Build history of the part. All positions in model axes, mm. Coordinates: 2 decimals unless noted, no trailing zeros. Order: outer loops, then holes, each group sorted by start corner. A loop starts at its lowest first (then second) coordinate and runs counter-clockwise, first axis right, second up. Notation, with made-up numbers: (-16, -36) - (-2, -36) arc R36 cw to (-2, -2) - close; hole circle Ø10 at (-12.5, -4). An arc over 180 degrees is marked (long way). One line per item, written item: value.
from build123d import *

# Parameters (mm, degrees)
SKETCH1_W           = 40.64
SKETCH1_H           = 50.673
SKETCH1_R           = 15.875
BOSS_EXTRUDE1_DEPTH = 6.35
CUT_EXTRUDE1_REACH  = 35.093
SKETCH2_R           = 2.665
FILLET1_R           = 2.54


with BuildPart() as part:
    # Sketch1 → Boss-Extrude1 (new body)
    with BuildSketch(Plane(origin=(0, 0, 0), x_dir=(1, 0, 0), z_dir=(0, 1, 0))):
        Rectangle(SKETCH1_W, SKETCH1_H)
        with Locations(Location((0, 0, 0), (0, 0, 270))):
            Circle(SKETCH1_R, mode=Mode.SUBTRACT)
    extrude(amount=BOSS_EXTRUDE1_DEPTH)

    # Sketch2 → Cut-Extrude1 (cut, up to next)
    with BuildSketch(Plane(origin=(0, 6.35, 0), x_dir=(1, 0, 0), z_dir=(0, 1, 0)), mode=Mode.PRIVATE) as cut_extrude1_sk1:
        with Locations(Location((-15.32, 20.3365, 0), (0, 0, 270))):
            Circle(SKETCH2_R)
    cut_extrude1_tool1 = extrude(cut_extrude1_sk1.sketch, amount=-CUT_EXTRUDE1_REACH, mode=Mode.PRIVATE) & part.part
    # Sketch2 → Cut-Extrude1 (cut, up to next)
    with BuildSketch(Plane(origin=(0, 6.35, 0), x_dir=(1, 0, 0), z_dir=(0, 1, 0)), mode=Mode.PRIVATE) as cut_extrude1_sk2:
        with Locations(Location((15.32, 20.3365, 0), (0, 0, 270))):
            Circle(SKETCH2_R)
    cut_extrude1_tool2 = extrude(cut_extrude1_sk2.sketch, amount=-CUT_EXTRUDE1_REACH, mode=Mode.PRIVATE) & part.part
    # Sketch2 → Cut-Extrude1 (cut, up to next)
    with BuildSketch(Plane(origin=(0, 6.35, 0), x_dir=(1, 0, 0), z_dir=(0, 1, 0)), mode=Mode.PRIVATE) as cut_extrude1_sk3:
        with Locations(Location((15.32, -20.3365, 0), (0, 0, 270))):
            Circle(SKETCH2_R)
    cut_extrude1_tool3 = extrude(cut_extrude1_sk3.sketch, amount=-CUT_EXTRUDE1_REACH, mode=Mode.PRIVATE) & part.part
    # Sketch2 → Cut-Extrude1 (cut, up to next)
    with BuildSketch(Plane(origin=(0, 6.35, 0), x_dir=(1, 0, 0), z_dir=(0, 1, 0)), mode=Mode.PRIVATE) as cut_extrude1_sk4:
        with Locations(Location((-15.32, -20.3365, 0), (0, 0, 270))):
            Circle(SKETCH2_R)
    cut_extrude1_tool4 = extrude(cut_extrude1_sk4.sketch, amount=-CUT_EXTRUDE1_REACH, mode=Mode.PRIVATE) & part.part
    add(cut_extrude1_tool1.solids().sort_by_distance((-15.32, 6.35, -20.3365))[0], mode=Mode.SUBTRACT)
    add(cut_extrude1_tool2.solids().sort_by_distance((15.32, 6.35, -20.3365))[0], mode=Mode.SUBTRACT)
    add(cut_extrude1_tool3.solids().sort_by_distance((15.32, 6.35, 20.3365))[0], mode=Mode.SUBTRACT)
    add(cut_extrude1_tool4.solids().sort_by_distance((-15.32, 6.35, 20.3365))[0], mode=Mode.SUBTRACT)

    # Fillet1
    fillet1_edges = [part.edges().sort_by_distance(p)[0] for p in [
        (20.32, 3.175, 25.3365),
        (-20.32, 3.175, 25.3365),
        (-20.32, 3.175, -25.3365),
        (20.32, 3.175, -25.3365),
    ]]
    fillet(fillet1_edges, radius=FILLET1_R)


solid = part.part
1. Two-plate mould, pull along Z, no slides. Class faces 1 (the face through (-19.6, 3.22, 24.57)), 2 (the face through (-17.92, 3.22, 19.76)), 3 (the face through (-20.32, 3, 0)): pulls with the +Z half, pulls with the -Z half, needs draft (parallel to the pull), parting line crosses it, or undercut.
Values found:
face 1: pulls with the +Z half
face 2: undercut
face 3: needs draft
2. Probe line 1 along X through (y, z) = (2, 19); line 2 along X through (y, z) = (4.25, 20); line 3 along Z through (x, y) = (-13.5, 4.75). List the from-to ranges inside material, lowest first.
Values found:
line 1: x = -20.32 to -17.63, -13.01 to 13.01, 17.63 to 20.32
line 2: x = -20.32 to -17.96, -12.68 to 12.68, 17.96 to 20.32
line 3: z = -25.34 to -22.28, -18.39 to -8.35, 8.35 to 18.39, 22.28 to 25.34
3. Band-saw the part on B-B, the plane y = 3.75. Count the separate pieces of the cut face and the enclosed holes in it, and give its area (3 significant figures).
Values found:
separate pieces: 1
enclosed holes: 5
area: 1,170 mm2
4. Band-saw the part on D-D, the plane z = 18.5. Give the cut face in (x, y), and give its area (3 significant figures).
Values found:
outline: (-20.32, 0) - (-17.25, 0) - (-17.25, 6.35) - (-20.32, 6.35) - close; (-13.39, 0) - (13.39, 0) - (13.39, 6.35) - (-13.39, 6.35) - close; (17.25, 0) - (20.32, 0) - (20.32, 6.35) - (17.25, 6.35) - close
area: 209 mm2
5. Flat gauge pin, fed straight in: P1, Ø19, axis at x = 0, z = 0, coming from the -Y side. Where does the tip first touch, or does it go through?
Values found:
P1: passes through
6. Band-saw the part on C-C, the plane z = 0. Give the cut face in (x, y) (3 decimals).
Values found:
outline: (-20.32, 0) - (-15.875, 0) - (-15.875, 6.35) - (-20.32, 6.35) - close; (15.875, 0) - (20.32, 0) - (20.32, 6.35) - (15.875, 6.35) - close
